CAD build for the part. Positions are in the model's coordinates, mm. Give positions to 0.01 mm unless a question says otherwise; leave off trailing zeros. Write each loop counter-clockwise with the first axis right and the second up, starting at its lowest first coordinate (ties: lowest second). Pieces come first, ordered by that corner, then holes. Notation, with made-up numbers: M 66,8 L 102,8 A9 ccw 102,22 Z; hole C 73,-14 d11. An arc over 180 degrees is marked long. One line per question, with ' | ' between items. Start each with the question number.
1. Cut at C-C, the plane z = 0.35. Write the cut outline in (x, y), then the cut area to 3 significant figures.
2. Cut at A-A, the plane x = 0. Write the cut outline in (y, z).
3. Flat gauge pin, fed straight in: pin 1 (8 mm diameter, centred on x = -30, y = 1, fed in from +Z). Where does the tip first touch, or does it go through?
4. Wall check: L1, parallel to Y at x = 0, z = 1.25; L2, parallel to Y at x = 0, z = 2.2; L3, parallel to Y at x = 18, z = 1.6. Give the ranges that are in metal, low to high.
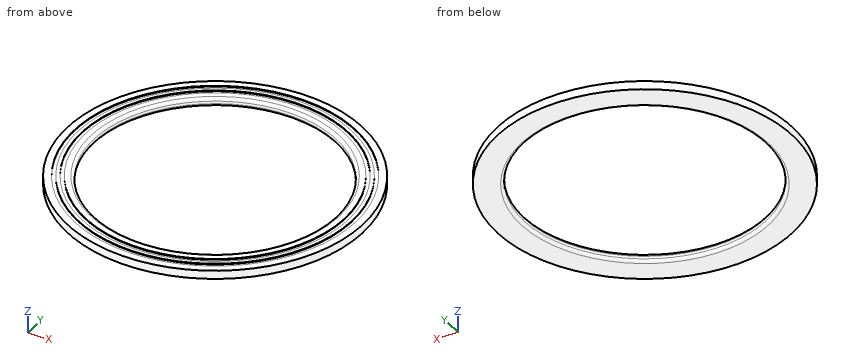
```python
from build123d import *

# Parameters (mm, degrees)
F0_R     = 40.5
F0_R_2   = 33.15
F1_DEPTH = 2.3
F2_R     = 0.8
F3_R     = 38.5
F3_R_2   = 37.5
F3_R_3   = 36.5
F3_R_4   = 35.5
F4_DEPTH = 0.2


with BuildPart() as f1:
    # F0 (on Top) → F1 (new body)
    with BuildSketch(Plane.XY):
        Circle(F0_R)
        Circle(F0_R_2, mode=Mode.SUBTRACT)
    extrude(amount=F1_DEPTH)

    # F2
    f2_edges = [f1.edges().sort_by_distance(p)[0] for p in [
        (-33.15, 0, 2.3),
        (-33.15, 0, 0),
    ]]
    fillet(f2_edges, radius=F2_R)

    # F3 (on face) → F4 (cut)
    with BuildSketch(Plane.XY.offset(2.3)):
        Circle(F3_R)
        Circle(F3_R_2, mode=Mode.SUBTRACT)
        Circle(F3_R_3)
        Circle(F3_R_4, mode=Mode.SUBTRACT)
    extrude(amount=-F4_DEPTH, mode=Mode.SUBTRACT)


solid = f1.part
```
Here are the results:
1) outline: C 0,0 d81; hole C 0,0 d66.58 | area: 1,670 mm^2
2) outline: M -40.5,0 L -33.95,0 A0.8 ccw -33.15,0.8 L -33.15,1.5 A0.8 ccw -33.95,2.3 L -35.5,2.3 L -35.5,2.1 L -36.5,2.1 L -36.5,2.3 L -37.5,2.3 L -37.5,2.1 L -38.5,2.1 L -38.5,2.3 L -40.5,2.3 Z; M 33.15,0.8 A0.8 ccw 33.95,0 L 40.5,0 L 40.5,2.3 L 38.5,2.3 L 38.5,2.1 L 37.5,2.1 L 37.5,2.3 L 36.5,2.3 L 36.5,2.1 L 35.5,2.1 L 35.5,2.3 L 33.95,2.3 A0.8 ccw 33.15,1.5 Z
3) pin 1: z = 2.3
4) L1: -40.5 to -33.15, 33.15 to 40.5 | L2: -40.5 to -38.5, -37.5 to -36.5, -35.5 to -33.56, 33.56 to 35.5, 36.5 to 37.5, 38.5 to 40.5 | L3: -36.28 to -27.84, 27.84 to 36.28
